The listing builds one solid part. Answer for the finished solid, in the listing's coordinates (mm). Coordinates: 2 decimals unless noted, no trailing zeros. Order: outer loops, then holes, each group sorted by start corner. A loop starts at its lowest first (then second) coordinate and runs counter-clockwise, first axis right, second up. Notation, with made-up numbers: (82, -26) - (101, -26) arc R35 ccw to (101, 12) - close; hole circle Ø6 at (-33, -26.5). An arc over 180 degrees is marked (long way). Use one line per item in the form item = value. Start each with the question number.
Item 1: The mould has two halves that part along Y. Classify faces 1 (the cylindrical face through (20.6, 30.5, -12.6)), 2 (the cylindrical face through (11.02, -8.67, -39.05)), 3 (the flat face through (1, -12, -35)): released by +Y, released by -Y, zero draft, split by the parting line, or undercut.
Item 2: Each of these flat-tipped pins is pushed along its axis until it touches: pin 1 Ø1.5 at (x, y) = (19.5, 6) entering from +Z; pin 2 Ø12 at (x, z) = (6.5, 25) entering from +Y; pin 3 Ø3 at (x, y) = (4.5, -5.5) entering from +Z. Where does it stop, or does it pass through?
Item 3: Section D-D, the plane x = 4.5 is taken. Write down the section's boundary in (y, z), and give its area (3 significant figures).
Item 4: Consider line 1 along Y through (x, z) = (14.75, -27); line 2 along Y through (x, z) = (18.5, 24.5); line 3 along Z through (x, y) = (14.75, -5.5). Determine where each line is inside the solid, lowest interval first. Write a range as [from, to].
Item 5: Section A-A, the plane z = 0 is taken. Write down the section's boundary in (x, y).
Item 6: Section C-C, the plane x = 16.25 is taken. Write down the section's boundary in (y, z), and give its area (3 significant figures).
from build123d import *

# Parameters (mm, degrees)
FILLET1_R = 1.5
FILLET2_R = 0.8
FILLET3_R = 0.4


with BuildPart() as part:
    # Sketch1 → Revolve1 (revolve)
    with BuildSketch(Plane.XY):
        Polygon((22, 33), (22, 40), (1, 40), (1, 36.267672581), (19.5318921, 33), align=None)
    revolve(axis=Axis((0, 0, 0), (1, 0, 0)))

    # Fillet1
    fillet1_edges = [part.edges().sort_by_distance(p)[0] for p in [
        (22, -40, 0),
    ]]
    fillet(fillet1_edges, radius=FILLET1_R)

    # Fillet2
    fillet2_edges = [part.edges().sort_by_distance(p)[0] for p in [
        (1, -40, 0),
    ]]
    fillet(fillet2_edges, radius=FILLET2_R)

    # Fillet3
    fillet3_edges = [part.edges().sort_by_distance(p)[0] for p in [
        (22, -33, 0),
        (1, -36.267672581, 0),
    ]]
    fillet(fillet3_edges, radius=FILLET3_R)


solid = part.part
Response:
q1.face_1 = undercut
q1.face_2 = split by the parting line
q1.face_3 = zero draft
q2.pin_1 = 39.65
q2.pin_2 = 35.2
q2.pin_3 = 39.8
q3.outline = circle Ø80 at (0, 0); hole circle Ø71.3 at (0, 0)
q3.area = 1,030 mm2
q4.line_1 = [-29.51, -20.4], [20.4, 29.51]
q4.line_2 = [-31.62, -22.38], [22.38, 31.62]
q4.line_3 = [-39.62, -33.39], [33.39, 39.62]
q5.outline = (1, -39.2) arc R0.8 ccw to (1.8, -40) - (20.5, -40) arc R1.5 ccw to (22, -38.5) - (22, -33.4) arc R0.4 ccw to (21.6, -33) - (19.53, -33) - (1.33, -36.21) arc R0.4 ccw to (1, -36.6) - close; (1, 36.6) arc R0.4 ccw to (1.33, 36.21) - (19.53, 33) - (21.6, 33) arc R0.4 ccw to (22, 33.4) - (22, 38.5) arc R1.5 ccw to (20.5, 40) - (1.8, 40) arc R0.8 ccw to (1, 39.2) - close
q6.outline = circle Ø80 at (0, 0); hole circle Ø67.16 at (0, 0)
q6.area = 1,480 mm2
